Autodesk Inventor part; units mm, degrees
ref_plane "Work Plane6" through (31.5, 0, 627) normal (1, 0, 0) x (0, 1, 0)
ref_plane "Work Plane7" through (31, 0, 0) normal (1, 0, 0) x (0, 1, 0)
ref_plane "Work Plane8" through (-0.7293, 31.4916, 0) normal (0, -0.3387, -0.9409) x (-1, 0, 0)
sketch "Sketch1" plane through (0, 0, 0) normal (0, 0, 1) x (1, 0, 0)
  circle A0 centre (0, 0) radius 31.5
  circle A1 centre (0, 0) radius 27.5
  dimension "d0" = 63
  dimension "d2" = 4
extrude "tube" add sketch "Sketch1" along normal blind 627
sketch "Sketch15" plane through (0, 0, 627) normal (0, 0, 1) x (1, 0, 0)
  circle A0 centre (0, 0) radius 27.5
  circle A1 centre (0, 0) radius 31.5
  point P0 (31.5, 0)
ref_plane "Work Plane6" through (31.5, 0, 627) normal (1, 0, 0) x (0, 1, 0)
ref_plane "Work Plane7" through (31, 0, 0) normal (1, 0, 0) x (0, 1, 0)
sketch "Sketch19" plane through (31, 0, 0) normal (1, 0, 0) x (0, 1, 0)
  line L0 (-10, 0) -> (10, 0)
  line L1 (10, 0) -> (10, 100)
  line L2 (10, 100) -> (-10, 100)
  line L3 (-10, 100) -> (-10, 0)
  point P0 (0, 0)
  point P1 (0, 0)
  dimension "d67" = 20
  dimension "d68" = 100
extrude "flatFaceYellow" cut sketch "Sketch19" along normal blind 25.4
sketch "Sketch21" plane through (0, 0, 0) normal (0, 0, -1) x (-1, 0, 0)
  line L0 (-31, 5.5902) -> (-31, -5.5902)
  arc A0 (-31, -5.5902) -> (-31, 5.5902) centre (0, 0) ccw
  circle A1 centre (0, 0) radius 27.5
  line L1 (0.7293, 31.4916) -> (30.8537, 31.4916) construction
ref_plane "Work Plane8" through (-0.7293, 31.4916, 0) normal (0, -0.3387, -0.9409) x (-1, 0, 0)
sketch "Sketch22" plane through (-0.7293, 31.4916, 0) normal (0, -0.3387, -0.9409) x (-1, 0, 0)
  line L0 (-34.8075, -84.5558) -> (31.7452, -84.5558)
  line L1 (31.7452, -84.5558) -> (31.7452, 8.8585)
  line L2 (31.7452, 8.8585) -> (-34.8075, 8.8585)
  line L3 (-34.8075, 8.8585) -> (-34.8075, -84.5558)
  point P0 (-0.7293, -29.6298)
extrude "angledEnd" cut sketch "Sketch22" along normal blind 25.4
sketch "Sketch23" plane through (31, 0, 0) normal (1, 0, 0) x (0, 0, -1)
  line L0 (-13.3502, -5.5902) -> (-100, -5.5902)
  circle A0 centre (-80, 0) radius 3.2074
  circle A1 centre (-40, 0) radius 3.2074
  point P0 (0, 0)
  dimension "d89" = 80
  dimension "d92" = 40
hole "Hole3" at (31, 0, 80) at (31, 0, 40) direction (-1, 0, 0) diameter 2 end through all
properties part number "2p5vss" material "PVC-Piping"
Here's how the part is built. I have some questions about the finished solid (model axes, mm). Give positions to 0.01 mm unless a question says otherwise; leave off trailing zeros. Order: outer loops, then holes, each group sorted by start corner. A loop starts at its lowest first (then second) coordinate and runs counter-clockwise, first axis right, second up. Notation, with made-up numbers: M 32,-20.5 L 37,-20.5 A28 ccw 37,6.5 Z; hole C 23,-27.5 d10. An arc over 180 degrees is marked long. Use a Markdown table: item, result. Add a question column.
1. For pin 1 Ø3.5 at (y, z) = (-2.5, 42.5) entering from +X; pin 2 Ø4 at (x, z) = (-6, 426.5) entering from -Y (3 decimals); pin 3 Ø2 at (x, z) = (-19.5, 405) entering from -Y, each with a flat end and sliding along its axis, tell me the tip position at first contact or that it passes through.
2. Suppose I cut it at A-A (y = 11.5). List the corners of the cut face in (x, z) for me, and give its area (3 significant figures).
3. Suppose I cut it at B-B (z = 361). List the corners of the cut face in (x, y) for me.
4. Suppose I cut it at C-C (y = -18). List the corners of the cut face in (x, z) for me, and give its area (3 significant figures).
5. I need wall thicknesses on probe 1 along Y at (x, z) = (1, 82.5); probe 2 along X at (y, z) = (-2.5, 545); probe 3 along X at (y, z) = (-1.5, 102). Which ranges of each line are inside material? Lowest first, please. Write a range as from..to.
6. If we mould it in two halves opening along X, with no side actions, what happens to faces 1 (the cylindrical face through (-4.101, -31.232, 309.111)), 2 (the flat face through (0, -28, 627)), 3 (the cylindrical face through (-5.961, 26.846, 309.824)), 4 (the flat face through (31, 0, 55))? For each: +X half, -X half, draft (parallel to the pull), parting line (faces both ways), or undercut.
Results list:
| question | item | result |
|---|---|---|
| 1 | pin 1 | stops at x = 31 |
| 1 | pin 2 | stops at y = -31.245 |
| 1 | pin 3 | stops at y = -25.5 |
| 2 | outline | M -29.33,7.2 L -24.98,7.2 L -24.98,627 L -29.33,627 Z; M 24.98,7.2 L 29.33,7.2 L 29.33,627 L 24.98,627 Z |
| 2 | area | 5,390 mm² |
| 3 | outline | C 0,0 d63; hole C 0,0 d55 |
| 4 | outline | M -25.85,17.82 L -20.79,17.82 L -20.79,627 L -25.85,627 Z; M 20.79,17.82 L 25.85,17.82 L 25.85,627 L 20.79,627 Z |
| 4 | area | 6,160 mm² |
| 5 | probe 1 | y = -31.48..-27.48, 27.48..31.48 |
| 5 | probe 2 | x = -31.4..-27.39, 27.39..31.4 |
| 5 | probe 3 | x = -31.46..-27.46, 27.46..31.46 |
| 6 | face 1 | parting line |
| 6 | face 2 | draft |
| 6 | face 3 | undercut |
| 6 | face 4 | +X half |
